Can you work these out from the model? Positions are in its coordinate system, mm. A direction names the side the tool comes from. Round coordinates to 2 decimals unless told otherwise and drop trailing zeros. Loops run counter-clockwise (first coordinate to the right, second up) from the corner with the lowest first, then second, coordinate; pieces in that order, holes last. Notation, with made-up numbers: (85.25, 10) -> (115.25, 10) arc R4 ccw to (115.25, 16) -> close; hole circle Ø11 at (-36, 52.5). An arc over 180 degrees is marked (long way). Answer as a JSON object with one key per item and string values.
```python
from build123d import *

# Parameters (mm, degrees)
BOSS_EXTRUDE1_DEPTH = 10.5
BOSS_EXTRUDE2_DEPTH = 42
CUT_REVOLVE1_ANGLE  = 180.0000000000004
CHAMFER1_SIZE       = 6
CHAMFER2_SIZE       = 2
CUT_EXTRUDE2_DEPTH  = 1
BOSS_EXTRUDE3_START = 6.5
BOSS_EXTRUDE3_DEPTH = 6.5
CHAMFER3_SIZE       = 1
SKETCH10_R          = 1.45
CUT_EXTRUDE6_DEPTH  = 10
SKETCH11_R          = 1.45
CUT_EXTRUDE7_DEPTH  = 72.20568797504873
MIRROR1_START       = 2
MIRROR1_DEPTH       = 17.247474683
SKETCH12_R          = 10.999999999999998
CUT_EXTRUDE8_DEPTH  = 5.25
SKETCH13_R          = 0.7500000000000007
SKETCH13_R_2        = 0.7499999999999987
SKETCH13_R_3        = 0.75
SKETCH13_R_4        = 0.7500000000000037
CUT_EXTRUDE9_DEPTH  = 3.25
SKETCH14_R          = 4.999999999999999
CUT_EXTRUDE10_DEPTH = 1.5
CUT_EXTRUDE11_DEPTH = 23.5


# Read off the part's stored shape, not the designer's step: Mirror1
with BuildPart() as part:
    # Sketch1 → Boss-Extrude1 (new body)
    with BuildSketch(Plane(origin=(0, 0, 0), x_dir=(1, 0, 0), z_dir=(0, 1, 0))):
        Polygon((-35, 0), (35, 0), (35, -14.497474683058336), (14.497474683058336, -35), (-14.497474683058336, -35), (-35, -14.497474683058334), align=None)
    extrude(amount=BOSS_EXTRUDE1_DEPTH)

    # Sketch2 → Boss-Extrude2 (add)
    with BuildSketch(Plane(origin=(0, 10.5, 0), x_dir=(1, 0, 0), z_dir=(0, 1, 0))):
        Polygon((-14.5, -32.5), (14.5, -32.49999999999999), (14.5, -23.499999999999993), (-14.5, -23.499999999999993), align=None)
    extrude(amount=BOSS_EXTRUDE2_DEPTH)

    # Sketch3 → Cut-Revolve1 (revolve, cut)
    with BuildSketch(Plane(origin=(0, 0, 0), x_dir=(-1, 0, 0), z_dir=(0, 0, -1))):
        Polygon((-27.000000000000004, 0), (-27.000000000000004, 3), (-29, 2.999999999999999), (-30.000000000000004, 4), (-30.000000000000004, 6.5), (-29, 7.500000000000001), (0, 7.5), (0, 0), align=None)
    revolve(axis=Axis((0, 0, 0), (0, -1, 0)), revolution_arc=CUT_REVOLVE1_ANGLE, mode=Mode.SUBTRACT)

    # Chamfer1
    chamfer1_edges = [part.edges().sort_by_distance(p)[0] for p in [
        (-14.5, 52.5, 27.999999999999996),
        (14.5, 52.5, 27.999999999999993),
    ]]
    chamfer(chamfer1_edges, length=CHAMFER1_SIZE)

    # Chamfer2
    # the kernel refuses this chamfer: 2 mm, written as the material it takes off along each edge
    with BuildSketch(Plane(origin=(38.63690895970556, 10.5, 10.860565723352778), x_dir=(-0.7068394360706735, 0.02749587661058652, -0.7068394360706735), z_dir=(-0.7071067811865476, 0, 0.7071067811865476)), Plane(origin=(-10.860565723352778, 10.5, 38.63690895970556), x_dir=(0.7068394360706735, 0.02749587661058652, -0.7068394360706735), z_dir=(-0.7071067811865476, 0, -0.7071067811865476))) as chamfer2_piece_1:
        Polygon((CHAMFER2_SIZE * 0.999621916911, CHAMFER2_SIZE * 0.0274958766106), (-CHAMFER2_SIZE * 0.0274958766106, CHAMFER2_SIZE * 0.999621916911), (0, 0), align=None)
    extrude(amount=39.28168131798029, mode=Mode.SUBTRACT)
    with BuildSketch(Plane(origin=(35, 10.5, -5.14336597593182), x_dir=(-0.9996219169112968, 0.02749587661058651, 0), z_dir=(0, 0, 1)), Plane(origin=(-35, 10.5, 19.640840658990157), x_dir=(0.9996219169112968, 0.02749587661058651, 0), z_dir=(0, 0, -1))) as chamfer2_piece_2:
        Polygon((CHAMFER2_SIZE * 0.999621916911, CHAMFER2_SIZE * 0.0274958766106), (-CHAMFER2_SIZE * 0.0274958766106, CHAMFER2_SIZE * 0.999621916911), (0, 0), align=None)
    extrude(amount=24.78420663492198, mode=Mode.SUBTRACT)
    with BuildSketch(Plane(origin=(14.5, 10.5, 32.49999999999999), x_dir=(-0.9996219169112968, 0, 0.027495876610585623), z_dir=(0, 1, 0))) as chamfer2_piece_3:
        Polygon((CHAMFER2_SIZE * 0.999621916911, -CHAMFER2_SIZE * 0.0274958766106), (-CHAMFER2_SIZE * 0.0274958766106, -CHAMFER2_SIZE * 0.999621916911), (0, 0), align=None)
    extrude(amount=41.14336597593182, mode=Mode.SUBTRACT)
    with BuildSketch(Plane(origin=(-14.5, 10.5, 32.5), x_dir=(-0.02749587661058651, 0, -0.9996219169112968), z_dir=(0, 1, 0))) as chamfer2_piece_4:
        Polygon((CHAMFER2_SIZE * 0.999621916911, -CHAMFER2_SIZE * 0.0274958766106), (-CHAMFER2_SIZE * 0.0274958766106, -CHAMFER2_SIZE * 0.999621916911), (0, 0), align=None)
    extrude(amount=41.14336597593182, mode=Mode.SUBTRACT)
    with BuildSketch(Plane(origin=(19.640840658990157, 10.5, 35), x_dir=(0, 0.02749587661058651, -0.9996219169112968), z_dir=(-1, 0, 0))) as chamfer2_piece_5:
        Polygon((CHAMFER2_SIZE * 0.999621916911, CHAMFER2_SIZE * 0.0274958766106), (-CHAMFER2_SIZE * 0.0274958766106, CHAMFER2_SIZE * 0.999621916911), (0, 0), align=None)
    extrude(amount=39.281681317980315, mode=Mode.SUBTRACT)

    # Sketch5 → Cut-Extrude2 (cut)
    with BuildSketch(Plane.XZ.offset(-7.5)):
        with BuildLine():
            Line((24, 8.82e-15), (-24, 0))
            ThreePointArc((-24, 0), (-23.247716404991003, 1.9964484090504302), (-21.365000000000002, 3))
            Line((-21.365000000000002, 3), (-12.000000000000002, 4.147))
            Line((-12.000000000000002, 4.147), (-6.125000000000002, 4.147000000000001))
            ThreePointArc((-6.125000000000002, 4.147000000000001), (-4.710786437626908, 4.732786437626906), (-4.125000000000002, 6.146999999999999))
            Line((-4.125000000000002, 6.146999999999999), (-4.125000000000002, 12.022))
            Line((-4.125000000000002, 12.022), (-2.9780000000000033, 21.387))
            ThreePointArc((-2.9780000000000033, 21.387), (1.8e-16, 24.365000000000002), (2.9780000000000033, 21.387))
            Line((2.9780000000000033, 21.387), (4.125000000000002, 12.022))
            Line((4.125000000000002, 12.022), (4.125000000000002, 6.146999999999999))
            ThreePointArc((4.125000000000002, 6.146999999999999), (4.710786437626908, 4.732786437626905), (6.125000000000002, 4.147000000000001))
            Line((6.125000000000002, 4.147000000000001), (12.000000000000002, 4.147))
            Line((12.000000000000002, 4.147), (21.365000000000002, 3))
            ThreePointArc((21.365000000000002, 3), (23.247716404991003, 1.996448409050434), (24, 8.82e-15))
        make_face()
    extrude(amount=-CUT_EXTRUDE2_DEPTH, mode=Mode.SUBTRACT)

    # Sketch6 → Boss-Extrude3 (add)
    with BuildSketch(Plane.XZ.offset(-7.5).offset(BOSS_EXTRUDE3_START)):
        with BuildLine():
            Line((14.499935981026823, 3.8408145680472217), (12.000000000000002, 4.147))
            Line((12.000000000000002, 4.147), (6.125000000000002, 4.147))
            ThreePointArc((6.125000000000002, 4.147), (4.710786437626906, 4.732786437626904), (4.125000000000002, 6.146999999999999))
            Line((4.125000000000002, 6.146999999999999), (4.125000000000002, 12.022))
            Line((4.125000000000002, 12.022), (3.8208636103945306, 14.505206005802291))
            ThreePointArc((3.8208636103945306, 14.505206005802291), (10.599303543236797, 10.613894874094425), (14.499935981026823, 3.8408145680472217))
        make_face()
        with BuildLine():
            Line((-3.8208636103945306, 14.505206005802291), (-4.125000000000002, 12.022))
            Line((-4.125000000000002, 12.022), (-4.125000000000003, 6.146999999999999))
            ThreePointArc((-4.125000000000003, 6.146999999999999), (-4.710786437626908, 4.732786437626906), (-6.125000000000002, 4.147000000000001))
            Line((-6.125000000000002, 4.147000000000001), (-12.000000000000002, 4.147))
            Line((-12.000000000000002, 4.147), (-14.499935981026823, 3.8408145680472217))
            ThreePointArc((-14.499935981026823, 3.8408145680472217), (-10.599303543236797, 10.613894874094424), (-3.8208636103945306, 14.505206005802291))
        make_face()
    extrude(amount=-BOSS_EXTRUDE3_DEPTH)

    # Chamfer3
    chamfer3_edges = [part.edges().sort_by_distance(p)[0] for p in [
        (10.5993035432368, 7.5, 10.613894874094427),
        (-10.599303543236797, 7.5, 10.613894874094424),
    ]]
    chamfer(chamfer3_edges, length=CHAMFER3_SIZE)

    # Sketch10 → Cut-Extrude6 (cut)
    with BuildSketch(Plane(origin=(0, 0, 0), x_dir=(-1, 0, 0), z_dir=(0, 0, -1))):
        with Locations((-32.5, 5.249999999999999)):
            Circle(SKETCH10_R)
        with Locations(Location((32.5, 5.249999999999999, 0), (0, 0, 180))):
            Circle(SKETCH10_R)
    extrude(amount=-CUT_EXTRUDE6_DEPTH, mode=Mode.SUBTRACT)

    # Sketch11 → Cut-Extrude7 (cut, through all)
    with BuildSketch(Plane(origin=(0, 0, 2), x_dir=(-1, 0, 0), z_dir=(0, 0, -1))):
        with BuildLine():
            Line((-32.5, 7.499999999999998), (-35, 7.499999999999998))
            Line((-35, 7.499999999999998), (-35, 3.000000000000001))
            Line((-35, 3.000000000000001), (-32.5, 3.0000000000000004))
            ThreePointArc((-32.5, 3.0000000000000004), (-30.25, 5.249999999999999), (-32.5, 7.499999999999998))
        make_face()
        with Locations((-32.5, 5.249999999999999)):
            Circle(SKETCH11_R, mode=Mode.SUBTRACT)
    extrude(amount=-CUT_EXTRUDE7_DEPTH, mode=Mode.SUBTRACT)


with BuildPart() as cut_extrude7_kept_piece:
    # of the separate pieces the step leaves, the one the design keeps (cut_extrude7_pieces_kept)
    add(part.part.solids().sort_by_distance((15.563806793, 7.5, 3.710514534))[0])

    # Mirror1 outline → Mirror1 (cut)
    with BuildSketch(Plane.XY.offset(MIRROR1_START)):
        with BuildLine():
            Line((-32.5, 7.5), (-35, 7.5))
            Line((-35, 7.5), (-35, 3))
            Line((-35, 3), (-32.5, 3))
            ThreePointArc((-32.5, 3), (-30.25, 5.25), (-32.5, 7.5))
        make_face()
    extrude(amount=MIRROR1_DEPTH, mode=Mode.SUBTRACT)

    # Sketch12 → Cut-Extrude8 (cut)
    with BuildSketch(Plane(origin=(0, 0, 23.499999999999993), x_dir=(-1, 0, 0), z_dir=(0, 0, -1))):
        with Locations((0, 32.5)):
            Circle(SKETCH12_R)
    extrude(amount=-CUT_EXTRUDE8_DEPTH, mode=Mode.SUBTRACT)

    # Sketch13 → Cut-Extrude9 (cut)
    with BuildSketch(Plane(origin=(0, 0, 28.749999999999993), x_dir=(-1, 0, 0), z_dir=(0, 0, -1))):
        with Locations((0, 25.25)):
            Circle(SKETCH13_R)
        with Locations((-7.249999999999999, 32.49999999999999)):
            Circle(SKETCH13_R_2)
        with Locations((-8.9e-16, 39.75)):
            Circle(SKETCH13_R_3)
        with Locations((7.249999999999999, 32.50000000000001)):
            Circle(SKETCH13_R_4)
    extrude(amount=-CUT_EXTRUDE9_DEPTH, mode=Mode.SUBTRACT)

    # Sketch14 → Cut-Extrude10 (cut)
    with BuildSketch(Plane(origin=(0, 0, 28.749999999999993), x_dir=(-1, 0, 0), z_dir=(0, 0, -1))):
        with Locations((0, 32.5)):
            Circle(SKETCH14_R)
    extrude(amount=-CUT_EXTRUDE10_DEPTH, mode=Mode.SUBTRACT)

    # Sketch16 → Cut-Extrude11 (cut)
    with BuildSketch(Plane(origin=(0, 0, 0), x_dir=(-1, 0, 0), z_dir=(0, 0, -1))):
        with BuildLine():
            Line((-6.708203932499372, 10.500000000000002), (6.708203932499372, 10.500000000000002))
            ThreePointArc((6.708203932499372, 10.500000000000002), (1.41e-15, 9.5), (-6.708203932499372, 10.500000000000002))
        make_face()
    extrude(amount=-CUT_EXTRUDE11_DEPTH, mode=Mode.SUBTRACT)


solid = cut_extrude7_kept_piece.part
```
Q1. I want a section at B-B, the plane y = 36. Write out the boundary of the cut face in (x, z).
Determined:
{"outline": "(-14.5, 23.5) -> (-10.43, 23.5) -> (-10.43, 28.75) -> (-3.57, 28.75) -> (-3.57, 30.25) -> (3.57, 30.25) -> (3.57, 28.75) -> (10.43, 28.75) -> (10.43, 23.5) -> (14.5, 23.5) -> (14.5, 30.5) -> (12.5, 32.5) -> (-12.5, 32.5) -> (-14.5, 30.5) -> close"}
Q2. On a 3-axis mill with a long thin cutter (end or side, diameter ignored), from which of +Z, -Z, +X, -X, +Y, -Y can I reach the whole of each face in a straight line? I mean faces 4 (the flat face through (-9, 5, 4.147)), 5 (the cylindrical face through (0.594, 1.521, 26.993)), 6 (the cylindrical face through (0.163, 24.518, 30.352)). Say none if no direction works.
Determined:
{"face 4": "-Z, -Y", "face 5": "-Y", "face 6": "-Z"}
Q3. If I drill on L1, parallel to Y at x = 0, z = 31; L2, parallel to Y at x = 0, z = 29; L3, parallel to Y at x = 28, z = 3, over which ranges is the centre line in solid material (lowest first)? Write a range as [from, to].
Determined:
{"L1": "[0, 24.5], [26, 39], [40.5, 52.5]", "L2": "[0, 3], [7.5, 24.5], [26, 27.5], [37.5, 39], [40.5, 52.5]", "L3": "[0, 3], [7.5, 10.5]"}
Q4. I want a section at A-A, the plane y = 18. Write out the boundary of the cut face in (x, z), then the cut area to 3 significant figures.
Determined:
{"outline": "(-14.5, 23.5) -> (14.5, 23.5) -> (14.5, 30.5) -> (12.5, 32.5) -> (-12.5, 32.5) -> (-14.5, 30.5) -> close", "area": "257 mm²"}
Q5. I'm going to push flat-ended pins straight in: pin 1 (10 mm diameter, centred on x = -9.5, z = 19, fed in from -Y); pin 2 (8 mm diameter, centred on x = 0.5, z = 7.5, fed in from +Y); pin 3 (1.7 mm diameter, centred on x = 0, y = 25.25, fed in from +Z). Where does each tip first touch, or does it pass through?
Determined:
{"pin 1": "y = 7.5", "pin 2": "y = 9.94", "pin 3": "z = 32.5"}
Q6. We'd pull the mould along Z, two halves only. Please class faces 1 (the flat face through (13, 29, 32)), 2 (the flat face through (-34, 3, 9)), 3 (the conical face through (0.641, 7.34, 29.153)): pulls with the +Z half, pulls with the -Z half, needs draft (parallel to the pull), parting line crosses it, or undercut.
Determined:
{"face 1": "pulls with the +Z half", "face 2": "needs draft", "face 3": "undercut"}
